Geometry: final body of the model. Coordinates: model frame, mm. A direction names the side the tool comes from. Give positions to 0.01 mm unless a question says otherwise; leave off trailing zeros. Loops run counter-clockwise (first coordinate to the right, second up) from the corner with the lowest first, then second, coordinate; pieces in that order, holes last. Notation, with made-up numbers: (4.25, 61) -> (49.25, 61) arc R13 ccw to (49.25, 86) -> close; hole circle Ø2 at (-27.75, 86.25). An arc over 180 degrees is marked (long way). Answer in a Markdown table with one row per item. Add a question column.
1) Line query: line 1 (X direction, y = -17.5, z = 29.5); line 2 (Z direction, x = 0, y = -25); line 3 (Z direction, x = 0.5, y = -21). Output: solid intervals per line, ascending. Write a range as from..to.
2) Section query A-A (z = 12.5). Return the cut outline in (x, y) (3 decimals), plus the area to 3 significant figures.
3) Section query B-B (x = 0). Return the cut outline in (y, z) (3 decimals).
4) First-contact query: P1, Ø1.8, axis at x = 15, z = 29.5, coming from the -Y side; P2, Ø1, axis at x = -8.5, z = 30.5, coming from the +Y side; P3, Ø2, axis at x = 0, z = 8, coming from the +Y side (3 decimals). Flat tips, straight axial feed; report the tip coordinate or a pass-through.
5) Section query C-C (y = -1). Give the number of separate pieces and of enclosed holes in the cut face, plus the area to 3 significant figures.
6) Section query D-D (x = 15). Return the cut outline in (y, z) (3 decimals).
7) Draft query along Z for faces 1 (the cylindrical face through (-6.396, -17.405, -5.35)), 2 (the cylindrical face through (-10.77, -34.14, 31.5)), 3 (the cylindrical face through (-10.77, -34.14, -10.5)). Return one class per face: +Z half, -Z half, draft (parallel to the pull), parting line (faces both ways), or undercut.
8) Access query for faces 4 (the flat face through (-12.2, -1, 11)), 5 (the cylindrical face through (-10.77, -1.39, 31.5)), 6 (the flat face through (0, -1, 33)), 7 (the flat face through (0, -34, 33)), 8 (the cylindrical face through (-10.74, -36.77, -2.38)). Directions: +Z, -Z, +X, -X, +Y, -Y. A direction counts if a zero-diameter tool reaches every point of the face in a straight line with its end or side. Return the directions, or none.
```python
from build123d import *
from OCP.BRepFilletAPI import BRepFilletAPI_MakeChamfer

# Parameters (mm, degrees)
SKETCH1_W                       = 24.4
SKETCH1_H                       = 45
BOSS_EXTRUDE1_DEPTH             = 35.5
FILLET1_R                       = 5
SKETCH2_W                       = 35.6
SKETCH2_H                       = 50.6
BOSS_EXTRUDE2_DEPTH             = 15
CHAMFER2_SIZE                   = 6
CHAMFER2_SIZE2                  = 7.679649793
FILLET2_R                       = 3
SKETCH3_R                       = 11
BOSS_EXTRUDE3_DEPTH             = 4
BOSS_EXTRUDE5_START             = -38
SKETCH3_3_R                     = 11
BOSS_EXTRUDE5_DEPTH             = 2.5
M2X0_4_TAPPED_HOLE1_D           = 1.6
M2X0_4_TAPPED_HOLE1_CSINK_D     = 2.05
M2X0_4_TAPPED_HOLE1_CSINK_ANGLE = 90
M2X0_4_TAPPED_HOLE2_D           = 1.6
M2X0_4_TAPPED_HOLE2_CSINK_D     = 2.05
M2X0_4_TAPPED_HOLE2_CSINK_ANGLE = 90


with BuildPart() as part:
    # Sketch1 → Boss-Extrude1 (new body)
    with BuildSketch(Plane(origin=(0, 0, 0), x_dir=(1, 0, 0), z_dir=(0, 1, 0))):
        with Locations((0, -10.5)):
            Rectangle(SKETCH1_W, SKETCH1_H)
    extrude(amount=-BOSS_EXTRUDE1_DEPTH)

    # Fillet1
    fillet1_edges = [part.edges().sort_by_distance(p)[0] for p in [
        (-12.2, -17.75, -12),
        (12.2, -17.75, -12),
        (12.2, -17.75, 33),
        (-12.2, -17.75, 33),
    ]]
    fillet(fillet1_edges, radius=FILLET1_R)

    # Sketch2 → Boss-Extrude2 (add, symmetric)
    with BuildSketch(Plane(origin=(0, -17.75, 0), x_dir=(1, 0, 0), z_dir=(0, 1, 0))):
        with Locations((0, -13.3)):
            Rectangle(SKETCH2_W, SKETCH2_H)
    extrude(amount=BOSS_EXTRUDE2_DEPTH, both=True)

    # Chamfer2: one chamfer whose edges measure the first distance from different faces: ONE call of the kernel's chamfer builder (chamfer() names one face for all edges)
    chamfer2_edges_1 = [part.edges().sort_by_distance(p)[0] for p in [
        (-17.8, -17.75, -12),
        (17.8, -17.75, -12),
    ]]
    chamfer2_side_1 = [part.faces().sort_by_distance(p)[0] for p in [
        (0, -17.75, -12),
    ]]
    chamfer2_edges_2 = [part.edges().sort_by_distance(p)[0] for p in [
        (-17.8, -17.75, 38.6),
        (17.8, -17.75, 38.6),
    ]]
    chamfer2_side_2 = [part.faces().sort_by_distance(p)[0] for p in [
        (0, -17.75, 38.6),
    ]]
    chamfer2 = BRepFilletAPI_MakeChamfer(part.part.solid().wrapped)
    for e in chamfer2_edges_1:
        chamfer2.Add(CHAMFER2_SIZE, CHAMFER2_SIZE2, e.wrapped, chamfer2_side_1[0].wrapped)  # the first distance lies on this face
    for e in chamfer2_edges_2:
        chamfer2.Add(CHAMFER2_SIZE, CHAMFER2_SIZE2, e.wrapped, chamfer2_side_2[0].wrapped)  # the first distance lies on this face
    add(Compound.cast(chamfer2.Shape()), mode=Mode.REPLACE)

    # Fillet2
    fillet2_edges = [part.edges().sort_by_distance(p)[0] for p in [
        (17.8, -17.75, -4.320350207),
        (17.8, -17.75, 30.920350207),
        (-11.8, -17.75, 38.6),
        (11.8, -17.75, 38.6),
        (-17.8, -17.75, -4.320350207),
        (-17.8, -17.75, 30.920350207),
        (-11.8, -17.75, -12),
        (11.8, -17.75, -12),
    ]]
    fillet(fillet2_edges, radius=FILLET2_R)

    # Sketch3 → Boss-Extrude3 (add)
    with BuildSketch(Plane(origin=(0, 0, 0), x_dir=(1, 0, 0), z_dir=(0, 1, 0))):
        with Locations(Location((0, 0, 0), (0, 0, 270))):
            Circle(SKETCH3_R)
    extrude(amount=BOSS_EXTRUDE3_DEPTH)

    # Sketch3<3> → Boss-Extrude5 (add)
    with BuildSketch(Plane(origin=(0, 0, 0), x_dir=(1, 0, 0), z_dir=(0, 1, 0)).offset(BOSS_EXTRUDE5_START)):
        with Locations(Location((0, 0, 0), (0, 0, 270))):
            Circle(SKETCH3_3_R)
    extrude(amount=BOSS_EXTRUDE5_DEPTH)

    # M2x0.4 Tapped Hole1 (through all)
    with Locations(Plane(origin=(0, 4, 0), x_dir=(1, 0, 0), z_dir=(0, 1, 0))):
        with Locations((-5.656854249, 5.656854249), (0, 8), (5.656854249, 5.656854249), (8, 0), (5.656854249, -5.656854249), (0, -8), (-5.656854249, -5.656854249), (-8, 0)):
            CounterSinkHole(M2X0_4_TAPPED_HOLE1_D / 2, M2X0_4_TAPPED_HOLE1_CSINK_D / 2, counter_sink_angle=M2X0_4_TAPPED_HOLE1_CSINK_ANGLE)

    # M2x0.4 Tapped Hole2 (through all)
    with Locations(Plane(origin=(0, -2.75, 0), x_dir=(1, 0, 0), z_dir=(0, 1, 0))):
        with Locations((15, 4.5), (-15, 4.5), (-15, -12.5), (-15, -29.5), (-8.5, -35.8), (8.5, -35.8), (15, -29.5), (15, -12.5)):
            CounterSinkHole(M2X0_4_TAPPED_HOLE2_D / 2, M2X0_4_TAPPED_HOLE2_CSINK_D / 2, counter_sink_angle=M2X0_4_TAPPED_HOLE2_CSINK_ANGLE)


solid = part.part
```
Evaluation:
| question | item | result |
|---|---|---|
| 1 | line 1 | -17.8..-15.8, -14.2..14.2, 15.8..17.8 |
| 1 | line 2 | -12..-8.8, -7.2..7.2, 8.8..38.6 |
| 1 | line 3 | -12..-8.62, -7.38..7.38, 8.62..38.6 |
| 2 | outline | (-17.8, -32.75) -> (-15.8, -32.75) -> (-15.8, -2.975) -> (-16.025, -2.75) -> (-17.8, -2.75) -> close; (-14.2, -32.75) -> (-12.2, -32.75) -> (-12.2, -35.5) -> (12.2, -35.5) -> (12.2, -32.75) -> (14.2, -32.75) -> (14.2, -2.975) -> (13.975, -2.75) -> (12.2, -2.75) -> (12.2, 0) -> (-12.2, 0) -> (-12.2, -2.75) -> (-13.975, -2.75) -> (-14.2, -2.975) -> close; (15.8, -32.75) -> (17.8, -32.75) -> (17.8, -2.75) -> (16.025, -2.75) -> (15.8, -2.975) -> close |
| 2 | area | 1,110 mm² |
| 3 | outline | (-38, -11) -> (-35.5, -11) -> (-35.5, -12) -> (0, -12) -> (0, -11) -> (4, -11) -> (4, -9.025) -> (3.775, -8.8) -> (-38, -8.8) -> close; (-38, -7.2) -> (3.775, -7.2) -> (4, -6.975) -> (4, 6.975) -> (3.775, 7.2) -> (-38, 7.2) -> close; (-38, 8.8) -> (3.775, 8.8) -> (4, 9.025) -> (4, 11) -> (0, 11) -> (0, 33) -> (-2.75, 33) -> (-2.75, 38.6) -> (-32.75, 38.6) -> (-32.75, 33) -> (-35.5, 33) -> (-35.5, 11) -> (-38, 11) -> close |
| 4 | P1 | y = -32.75 |
| 4 | P2 | y = 0 |
| 4 | P3 | y = 3.975 |
| 5 | separate pieces | 1 |
| 5 | enclosed holes | 8 |
| 5 | area | 1,060 mm² |
| 6 | outline | (-32.75, -7.904) -> (-2.75, -7.904) -> (-2.75, -5.525) -> (-2.975, -5.3) -> (-32.75, -5.3) -> close; (-32.75, -3.7) -> (-2.975, -3.7) -> (-2.75, -3.475) -> (-2.75, 11.475) -> (-2.975, 11.7) -> (-32.75, 11.7) -> close; (-32.75, 13.3) -> (-2.975, 13.3) -> (-2.75, 13.525) -> (-2.75, 28.475) -> (-2.975, 28.7) -> (-32.75, 28.7) -> close; (-32.75, 30.3) -> (-2.975, 30.3) -> (-2.75, 30.525) -> (-2.75, 34.504) -> (-32.75, 34.504) -> close |
| 7 | face 1 | undercut |
| 7 | face 2 | +Z half |
| 7 | face 3 | -Z half |
| 8 | face 4 | +Z, -Z, -X, +Y |
| 8 | face 5 | +Z, -X, +Y |
| 8 | face 6 | +Z, +X, -X, +Y |
| 8 | face 7 | +Z, +X, -X, -Y |
| 8 | face 8 | -Y |
